Autodesk Inventor part; units mm, degrees
ref_plane "Work Plane1" through (0, 8.9795, -42.5) normal (0, 1, 0) x (-1, 0, 0)
ref_plane "YZ Plane" through (0, 0, 0) normal (1, 0, 0) x (0, 1, 0)
ref_plane "XY Plane" through (0, 0, 0) normal (0, 0, 1) x (1, 0, 0)
sketch "Sketch1" plane through (0, 0, 0) normal (1, 0, 0) x (0, 1, 0)
  line L0 (0, 0) -> (0, -85)
  line L1 (0, -85) -> (8, -85)
  line L2 (0, 0) -> (8, 0)
  line L3 (8, 0) -> (8, -14)
  line L4 (8, -85) -> (8, -71)
  line L5 (8, -14) -> (9, -14)
  line L6 (8, -71) -> (9, -71)
  arc A0 (10.5, -14.5) -> (10.5, -70.5) centre (267.5593, -42.5) ccw
  line L7 (8, -71) -> (10.555, -71)
  line L8 (8, -14) -> (10.555, -14)
  arc A1 (10.555, -14) -> (10.555, -71) centre (267.5473, -42.5) ccw
extrude "Extrusion1" add sketch "Sketch1" along normal mid plane 14
sketch "Sketch2" plane through (-7, 8, 0) normal (0, 1, 0) x (1, 0, 0)
  line L0 (0, 85) -> (0, 0)
  line L1 (0, 14.0338) -> (0, 5.5338)
  line L2 (14, 0) -> (14, 85)
  line L3 (14, 14.0338) -> (14, 5.5338)
  arc A0 (0, 5.5338) -> (14, 5.5338) centre (7, 7.1942) ccw
  line L4 (0, 5.5338) -> (0, 0)
  line L5 (0, 0) -> (14, 0)
  line L6 (14, 0) -> (14, 5.5338)
  point P0 (7, 0)
  dimension "d13" = 8.5
extrude "Extrusion2" cut sketch "Sketch2" against normal blind 14
sketch "Sketch3" plane through (-7, 8, -71) normal (0, 1, 0) x (1, 0, 0)
  line L0 (0, 0) -> (14, 0)
  line L1 (0, 0) -> (0, 14)
  arc A0 (14, 8.5) -> (0, 8.5) centre (7, 6.7955) ccw
  line L2 (0, 8.5) -> (0, 14)
  line L3 (0, 14) -> (14, 14)
  line L4 (14, 14) -> (14, 8.5)
  line L5 (14, -65.4662) -> (14, 14)
  line L6 (0, 14) -> (0, 8.5)
  line L7 (14, 8.5) -> (14, 14)
  line L8 (14, 14) -> (0, 14)
  line L9 (0, 8.5) -> (0, 14)
  line L10 (0, 14) -> (14, 14)
  line L11 (14, 14) -> (14, 8.5)
  line L12 (14, 14) -> (14, 0)
  arc A1 (14, 8.5) -> (0, 8.5) centre (7, 6.7955) ccw
  point P0 (7, -71)
extrude "Extrusion3" cut sketch "Sketch3" against normal blind 14 contours L1 L3 A0 | A0 L3 L4
sketch "Sketch4" plane through (-7, 8, -71) normal (0, 1, 0) x (1, 0, 0)
  arc A0 (14, 8.5) -> (0, 8.5) centre (7, 6.7955) ccw
  line L0 (7, 0.0396) -> (7, 3.0396)
  circle A1 centre (7, 9) radius 3
  point P0 (7, -71)
extrude "Extrusion4" cut sketch "Sketch4" against normal blind 14
sketch "Sketch5" plane through (-7, 8, -14) normal (0, 1, 0) x (1, 0, 0)
  circle A0 centre (7, -9) radius 3
  point P0 (7, -14)
extrude "Extrusion5" cut sketch "Sketch5" against normal blind 14
sketch "Sketch7" plane through (0, 0, -7.1942) normal (0, -1, 0) x (1, 0, 0)
  circle A0 centre (0, 2.1942) radius 3
  line L0 (0, -0.8058) -> (0, -3.8058)
  circle A1 centre (0, -72.8058) radius 3
  line L1 (0, -69.8058) -> (0, -66.8058)
  line L2 (0, -66.8058) -> (-5, -66.8058)
  line L3 (-5, -66.8058) -> (5, -66.8058)
  line L4 (-5, -66.8058) -> (5, -66.8058)
  line L5 (5, -66.8058) -> (5, -56.7258)
  line L6 (5, -56.7258) -> (-5, -56.7258)
  line L7 (-5, -56.7258) -> (-5, -66.8058)
  line L8 (0, -56.7258) -> (0, -56.2258)
  line L9 (-5, -56.2258) -> (5, -56.2258)
  line L10 (5, -56.2258) -> (5, -46.1458)
  line L11 (5, -46.1458) -> (-5, -46.1458)
  line L12 (-5, -46.1458) -> (-5, -56.2258)
  line L13 (0, -46.1458) -> (0, -45.6458)
  line L14 (-5, -45.6458) -> (5, -45.6458)
  line L15 (5, -45.6458) -> (5, -35.5658)
  line L16 (5, -35.5658) -> (-5, -35.5658)
  line L17 (-5, -35.5658) -> (-5, -45.6458)
  line L18 (0, -35.5658) -> (0, -35.0658)
  line L19 (-5, -35.0658) -> (5, -35.0658)
  line L20 (5, -35.0658) -> (5, -24.9858)
  line L21 (5, -24.9858) -> (-5, -24.9858)
  line L22 (-5, -24.9858) -> (-5, -35.0658)
  line L23 (0, -24.9858) -> (0, -24.4858)
  line L24 (-5, -24.4858) -> (5, -24.4858)
  line L25 (5, -24.4858) -> (5, -14.4058)
  line L26 (5, -14.4058) -> (-5, -14.4058)
  line L27 (-5, -14.4058) -> (-5, -24.4858)
  line L28 (0, -14.4058) -> (0, -13.9058)
  line L29 (-5, -13.9058) -> (5, -13.9058)
  line L30 (5, -13.9058) -> (5, -3.8058)
  line L31 (5, -3.8058) -> (-5, -3.8058)
  line L32 (-5, -3.8058) -> (-5, -13.9058)
  point P0 (0, 7.1942)
extrude "Extrusion6" cut sketch "Sketch7" against normal blind 1.5 contours L6 L5 L3 L2 L7 | L31 L30 L29 L32
sketch "Sketch8" plane through (0, 0, -7.1942) normal (0, -1, 0) x (1, 0, 0)
  line L0 (-5, -56.7258) -> (5, -56.7258)
  line L1 (0, -56.7258) -> (0, -56.2258)
  line L2 (-5, -56.2258) -> (5, -56.2258)
  line L3 (5, -56.2258) -> (5, -46.1458)
  line L4 (5, -46.1458) -> (-5, -46.1458)
  line L5 (-5, -46.1458) -> (-5, -56.2258)
  line L6 (0, -46.1458) -> (0, -45.6458)
  line L7 (-5, -45.6458) -> (5, -45.6458)
  line L8 (5, -45.6458) -> (5, -35.5658)
  line L9 (5, -35.5658) -> (-5, -35.5658)
  line L10 (-5, -35.5658) -> (-5, -45.6458)
  line L11 (0, -35.5658) -> (0, -35.0658)
  line L12 (-5, -35.0658) -> (5, -35.0658)
  line L13 (5, -35.0658) -> (5, -24.9858)
  line L14 (5, -24.9858) -> (-5, -24.9858)
  line L15 (-5, -24.9858) -> (-5, -35.0658)
  line L16 (0, -24.9858) -> (0, -24.4858)
  line L17 (-5, -24.4858) -> (5, -24.4858)
  line L18 (5, -24.4858) -> (5, -14.4058)
  line L19 (5, -14.4058) -> (-5, -14.4058)
  line L20 (-5, -14.4058) -> (-5, -24.4858)
  point P0 (0, 7.1942)
  dimension "d75" = 0.5
  dimension "d76" = 10.08
  dimension "d77" = 0.5
  dimension "d78" = 10.08
  dimension "d79" = 0.5
  dimension "d80" = 10.08
  dimension "d81" = 0.5
  dimension "d82" = 10.08
extrude "Extrusion7" cut sketch "Sketch8" against normal blind 1
sketch "Sketch9" plane through (0, 1.5, -7.1942) normal (0, -1, 0) x (1, 0, 0)
  line L0 (-5, -66.8058) -> (-5, -56.7258)
  line L1 (5, -56.7258) -> (5, -66.8058)
  line L2 (-5, -59.2658) -> (5, -59.2658)
  line L3 (-5, -64.2658) -> (5, -64.2658)
  line L4 (-5, -64.2658) -> (-5, -59.2658)
  line L5 (5, -64.2658) -> (5, -59.2658)
  line L6 (5, -64.2658) -> (5, -59.2658)
  point P0 (0, 7.1942)
extrude "Extrusion8" cut sketch "Sketch9" against normal blind 20
sketch "Sketch10" plane through (0, 1, -7.1942) normal (0, -1, 0) x (1, 0, 0)
  line L0 (-5, -56.2258) -> (-5, -46.1458)
  line L1 (5, -46.1458) -> (5, -56.2258)
  line L2 (-5, -53.6858) -> (5, -53.6858)
  line L3 (-5, -48.6858) -> (5, -48.6858)
  line L4 (5, -48.6858) -> (5, -53.6858)
  line L5 (-5, -48.6858) -> (-5, -53.6858)
  point P0 (0, 7.1942)
  dimension "d109" = 5
extrude "Extrusion9" cut sketch "Sketch10" against normal blind 20
sketch "Sketch11" plane through (0, 1, -7.1942) normal (0, -1, 0) x (1, 0, 0)
  line L0 (-5, -45.6458) -> (-5, -35.5658)
  line L1 (5, -35.5658) -> (5, -45.6458)
  line L2 (-5, -43.1058) -> (5, -43.1058)
  line L3 (-5, -38.1058) -> (5, -38.1058)
  line L4 (5, -38.1058) -> (5, -43.1058)
  line L5 (-5, -38.1058) -> (-5, -43.1058)
  point P0 (0, 7.1942)
extrude "Extrusion10" cut sketch "Sketch11" against normal blind 20
sketch "Sketch12" plane through (0, 1, -7.1942) normal (0, -1, 0) x (1, 0, 0)
  line L0 (-5, -35.0658) -> (-5, -24.9858)
  line L1 (5, -24.9858) -> (5, -35.0658)
  line L2 (-5, -32.5258) -> (5, -32.5258)
  line L3 (-5, -27.5258) -> (5, -27.5258)
  line L4 (5, -27.5258) -> (5, -32.5258)
  line L5 (-5, -27.5258) -> (-5, -32.5258)
  point P0 (0, 7.1942)
extrude "Extrusion11" cut sketch "Sketch12" against normal blind 20
sketch "Sketch13" plane through (0, 1, -7.1942) normal (0, -1, 0) x (1, 0, 0)
  line L0 (-5, -24.4858) -> (-5, -14.4058)
  line L1 (-5, -21.9458) -> (5, -21.9458)
  line L2 (-5, -16.9458) -> (5, -16.9458)
  line L3 (5, -16.9458) -> (5, -21.9458)
  line L4 (5, -14.4058) -> (5, -24.4858)
  line L5 (-5, -16.9458) -> (-5, -21.9458)
  point P0 (0, 7.1942)
extrude "Extrusion12" cut sketch "Sketch13" against normal blind 20
sketch "Sketch14" plane through (0, 1.5, -7.1942) normal (0, -1, 0) x (1, 0, 0)
  line L0 (-5, -13.9058) -> (-5, -3.8058)
  line L1 (5, -3.8058) -> (5, -13.9058)
  line L2 (-5, -11.3558) -> (5, -11.3558)
  line L3 (-5, -6.3558) -> (5, -6.3558)
  line L4 (5, -6.3558) -> (5, -11.3558)
  line L5 (-5, -6.772) -> (-5, -11.3558)
  line L6 (-5, -6.3558) -> (-5, -11.3558)
  point P0 (0, 7.1942)
extrude "Extrusion13" cut sketch "Sketch14" against normal blind 20
ref_plane "Work Plane1" through (0, 8.9795, -42.5) normal (0, 1, 0) x (-1, 0, 0)
sketch "Sketch24" plane through (5, 0, -74) normal (-1, 0, 0) x (0, 0, 1)
  line L0 (7.54, 1.5) -> (7.54, 10.0921)
  line L1 (2.54, 8) -> (3, 8)
  circle A0 centre (4.961, 4.75) radius 1
  line L2 (13.12, 1) -> (13.12, 9.6336)
  line L3 (18.12, 1) -> (18.12, 9.326)
  circle A1 centre (15.62, 5.3168) radius 1
  line L4 (23.7, 1) -> (23.7, 9.0972)
  line L5 (28.7, 1) -> (28.7, 8.9947)
  circle A2 centre (26.2398, 4.9841) radius 1
  line L6 (34.28, 1) -> (31.74, 1)
  circle A3 centre (36.749, 5.0486) radius 1
  line L7 (44.86, 1) -> (42.32, 1)
  circle A4 centre (47.3544, 5.3168) radius 1
  line L8 (60.45, 1.5) -> (60.45, 8)
  line L9 (55.45, 1.5) -> (55.45, 10.0911)
  circle A5 centre (57.95, 5.7956) radius 1
  point P0 (74, 0)
  point P1 (2.54, 1.5)
extrude "Extrusion14" cut sketch "Sketch24" along normal mid plane 52
sketch "Sketch25" plane through (7, 0, 0) normal (1, 0, 0) x (0, 0, -1)
  circle A0 centre (69.039, 4.75) radius 1
  circle A1 centre (58.38, 5.3168) radius 1
  circle A2 centre (47.7602, 4.9841) radius 1
  circle A3 centre (37.251, 5.0486) radius 1
  circle A4 centre (26.6456, 5.3168) radius 1
  circle A5 centre (16.05, 5.7956) radius 1
  circle A6 centre (16.05, 5.7956) radius 1.75
  circle A7 centre (26.6456, 5.3168) radius 1.75
  circle A8 centre (37.251, 5.0486) radius 1.75
  circle A9 centre (47.7602, 4.9841) radius 1.75
  circle A10 centre (58.38, 5.3168) radius 1.75
  circle A11 centre (69.039, 4.75) radius 1
  circle A12 centre (69.039, 4.75) radius 1.75
  point P0 (0, 0)
  dimension "d129" = 3.5
  dimension "d130" = 3.5
  dimension "d131" = 3.5
  dimension "d132" = 3.5
  dimension "d133" = 3.5
  dimension "d134" = 3.5
extrude "Extrusion15" cut sketch "Sketch25" against normal blind 5
properties part number "segurador das cordas" material "Steel"
The model under review builds one solid part; all positions refer to its coordinate system, in mm. A direction names the side the tool comes from. Round coordinates to 2 decimals unless told otherwise and drop trailing zeros. Order: outer loops, then holes, each group sorted by start corner. A loop starts at its lowest first (then second) coordinate and runs counter-clockwise, first axis right, second up. Notation, with made-up numbers: (30, 15.25) -> (68, 15.25) arc R8 cw to (68, 29.25) -> close; hole circle Ø1 at (51, 43.25). An arc over 180 degrees is marked (long way). Write item = value, one per line. Start each with the question number.
Item 1: Consider section A-A on x = 0. Count the separate pieces of the cut face and the enclosed holes in it, plus the area to 3 significant figures.
Item 2: Consider section B-B on z = -16.05. Write out the cut boundary in (x, y), plus the area to 3 significant figures.
Item 3: For line 1 along Z through (x, y) = (1, 8.5); line 2 along X through (y, z) = (4, -66.5); line 3 along Y through (x, z) = (4.25, -72), list the stretches that pass through material, from the lowest coordinate up.
Item 4: Mouldability with a two-part tool opening along Z and no side actions: class faces 6 (the face through (6, 9, -14)), 7 (the face through (5, 3, -49)), 8 (the face through (-0.65, 4.06, -2.07)), 9 (the face through (5.2, 0, -39.2)) as released by +Z, released by -Z, zero draft, split by the parting line, or undercut.
Item 5: Clearance check with flat-ended pins moving along their axes: pin 1 Ø5 at (x, z) = (-2, -15) entering from -Y; pin 2 Ø0.6 at (x, y) = (-6, 9.5) entering from +Z; pin 3 Ø1.3 at (x, z) = (0, -33.5) entering from -Y. State where each tip first meets the part, or that it passes through.
Item 6: For faces 1 (the face through (0, 5, -71.46)), 2 (the face through (0, 1.5, -20)), 3 (the face through (-6, 9, -14)), 4 (the face through (-5.986, 5.016, -57.426)), 5 (the face through (6.01, 6.98, -14.76)), list the 3-axis set-ups (+Z, -Z, +X, -X, +Y, -Y) from which the entire face can be reached by the end or side of a thin tool; tool diameter is ignored.
Item 7: Consider section C-C on z = -62. Write out the cut boundary in (x, y).
Item 8: Consider section D-D on z = -34. Write out the cut boundary in (x, y).
Conclusion:
q1.separate_pieces = 9
q1.enclosed_holes = 0
q1.area = 348 mm2
q2.outline = (-7, 0) -> (-5, 0) -> (-5, 4.8) -> (-7, 4.8) -> close; (-7, 6.8) -> (-5, 6.8) -> (-5, 10.34) -> (-7, 10.34) -> close; (5, 0) -> (7, 0) -> (7, 4.05) -> (5, 4.05) -> close; (5, 7.55) -> (7, 7.55) -> (7, 10.34) -> (5, 10.34) -> close
q2.area = 30.3 mm2
q3.line_1 = -66.46 to -60.88, -55.88 to -50.3, -45.3 to -39.72, -34.72 to -29.14, -24.14 to -18.55
q3.line_2 = -7 to -5, 5 to 7
q3.line_3 = 1.5 to 8
q4.face_6 = released by +Z
q4.face_7 = undercut
q4.face_8 = undercut
q4.face_9 = zero draft
q5.pin_1 = 1.5
q5.pin_2 = -14
q5.pin_3 = 1
q6.face_1 = +Y, -Y
q6.face_2 = -Y
q6.face_3 = +Z, +X, -X, +Y
q6.face_4 = +X, -X
q6.face_5 = +X
q7.outline = (-7, 0) -> (-5, 0) -> (-5, 1) -> (5, 1) -> (5, 0) -> (7, 0) -> (7, 9.72) -> (-7, 9.72) -> close
q8.outline = (-7, 0) -> (-5, 0) -> (-5, 1) -> (5, 1) -> (5, 0) -> (7, 0) -> (7, 9.12) -> (-7, 9.12) -> close
